```python
from build123d import *

# Parameters (mm, degrees)
CYLINDER024_R               = 7.5
CYLINDER024_DEPTH           = 2
CYLINDER012_R               = 3.15
CYLINDER012_DEPTH           = 43
CYLINDER011_R               = 2
CYLINDER011_DEPTH           = 39
CYLINDER013_R               = 2.55
CYLINDER013_DEPTH           = 6
BOX022_W                    = 1
BOX022_H                    = 7
BOX022_DEPTH                = 4
BOX023_W                    = 1
BOX023_H                    = 7
BOX023_DEPTH                = 4
CHAMFER003068012002016_SIZE = 3
BOX020_W                    = 7.8
BOX020_H                    = 3
BOX020_DEPTH                = 1
BOX018_W                    = 7.8
BOX018_H                    = 7
BOX018_DEPTH                = 1
BOX021_W                    = 5
BOX021_H                    = 4
BOX021_DEPTH                = 5
CHAMFER003068012002041_SIZE = 3
CHAMFER003068012002042_SIZE = 0.4
BOX017_W                    = 25
BOX017_H                    = 5
BOX017_DEPTH                = 24
CHAMFER003068012002002_SIZE = 4
BOX015_W                    = 24
BOX015_H                    = 20
BOX015_DEPTH                = 38
CHAMFER003068012002006_SIZE = 2
CHAMFER003068012002007_SIZE = 2
CHAMFER003068012002009_SIZE = 0.4
CYLINDER023_R               = 6
CYLINDER023_DEPTH           = 27
CHAMFER003068012002044_SIZE = 0.4
CHAMFER003068012002045_SIZE = 0.4


with BuildPart() as cylinder024:
    # Cylinder024 → Cylinder024 (new body)
    with BuildSketch(Plane(origin=(-15, 6, -12), x_dir=(1, 0, 0), z_dir=(0, 0, 1))):
        Circle(CYLINDER024_R)
    extrude(amount=CYLINDER024_DEPTH)


with BuildPart() as cylinder012:
    # Cylinder012 → Cylinder012 (new body)
    with BuildSketch(Plane(origin=(-15, 6, -11), x_dir=(1, 0, 0), z_dir=(0, 0, 1))):
        Circle(CYLINDER012_R)
    extrude(amount=CYLINDER012_DEPTH)


with BuildPart() as cylinder011:
    # Cylinder011 → Cylinder011 (new body)
    with BuildSketch(Plane(origin=(1, 13, -5), x_dir=(0, 0, 1), z_dir=(-1, 0, 0))):
        Circle(CYLINDER011_R)
    extrude(amount=CYLINDER011_DEPTH)


with BuildPart() as fusion001002012005:
    # Cylinder013 → Cylinder013 (new body)
    with BuildSketch(Plane(origin=(1, 13, -5), x_dir=(0, 0, 1), z_dir=(-1, 0, 0))):
        Circle(CYLINDER013_R)
    extrude(amount=CYLINDER013_DEPTH)

    # Fusion001002012005: union Cylinder011
    add(cylinder011.part)


with BuildPart() as cube022:
    # Box022 → Box022 (new body)
    with BuildSketch(Plane(origin=(-2.5, 0.5, 16.5), x_dir=(1, 0, 0), z_dir=(0, 0, 1))):
        with Locations((0.5, 3.5)):
            Rectangle(BOX022_W, BOX022_H)
    extrude(amount=BOX022_DEPTH)


with BuildPart() as chamfer003068012002016:
    # Box023 → Box023 (new body)
    with BuildSketch(Plane(origin=(-2.5, 0.5, 11), x_dir=(1, 0, 0), z_dir=(0, 0, 1))):
        with Locations((0.5, 3.5)):
            Rectangle(BOX023_W, BOX023_H)
    extrude(amount=BOX023_DEPTH)

    # Fusion001002012009: union Cube022
    add(cube022.part)

    # Chamfer003068012002016
    chamfer003068012002016_edges = [chamfer003068012002016.edges().sort_by_distance(p)[0] for p in [
        (-2, 0.5, 11),
        (-2, 7.5, 11),
        (-2, 0.5, 20.5),
        (-2, 7.5, 20.5),
    ]]
    chamfer(chamfer003068012002016_edges, length=CHAMFER003068012002016_SIZE)


with BuildPart() as chamfer003068012002016_1:
    # Chamfer003068012002016 placement: moved
    add(chamfer003068012002016.part.moved(Location((0, 0, 1.5))))


with BuildPart() as cube020:
    # Box020 → Box020 (new body)
    with BuildSketch(Plane(origin=(-18.9, -2, 28), x_dir=(1, 0, 0), z_dir=(0, 0, 1))):
        with Locations((3.9, 1.5)):
            Rectangle(BOX020_W, BOX020_H)
    extrude(amount=BOX020_DEPTH)


with BuildPart() as fusion001002012023:
    # Box018 → Box018 (new body)
    with BuildSketch(Plane(origin=(-18.9, 11, 28), x_dir=(1, 0, 0), z_dir=(0, 0, 1))):
        with Locations((3.9, 3.5)):
            Rectangle(BOX018_W, BOX018_H)
    extrude(amount=BOX018_DEPTH)

    # Fusion001002012023: union Cube020
    add(cube020.part)


with BuildPart() as chamfer003068012002042:
    # Box021 → Box021 (new body)
    with BuildSketch(Plane(origin=(-26, -5, -5), x_dir=(1, 0, 0), z_dir=(0, 0, 1))):
        with Locations((2.5, 2)):
            Rectangle(BOX021_W, BOX021_H)
    extrude(amount=BOX021_DEPTH)

    # Chamfer003068012002041
    chamfer003068012002041_edges = [chamfer003068012002042.edges().sort_by_distance(p)[0] for p in [
        (-23.5, -5, -5),
    ]]
    chamfer(chamfer003068012002041_edges, length=CHAMFER003068012002041_SIZE)

    # Chamfer003068012002042
    chamfer003068012002042_edges = [chamfer003068012002042.edges().sort_by_distance(p)[0] for p in [
        (-26, -5, -1),
        (-26, -3.5, -3.5),
        (-26, -3, 0),
        (-21, -5, -1),
        (-21, -3.5, -3.5),
        (-21, -3, 0),
    ]]
    chamfer(chamfer003068012002042_edges, length=CHAMFER003068012002042_SIZE)


with BuildPart() as chamfer003068012002002:
    # Box017 → Box017 (new body)
    with BuildSketch(Plane(origin=(-26, 11, 2), x_dir=(1, 0, 0), z_dir=(0, 0, 1))):
        with Locations((12.5, 2.5)):
            Rectangle(BOX017_W, BOX017_H)
    extrude(amount=BOX017_DEPTH)

    # Chamfer003068012002002
    chamfer003068012002002_edges = [chamfer003068012002002.edges().sort_by_distance(p)[0] for p in [
        (-13.5, 11, 2),
        (-13.5, 11, 26),
    ]]
    chamfer(chamfer003068012002002_edges, length=CHAMFER003068012002002_SIZE)


with BuildPart() as chamfer003068012002009:
    # Box015 → Box015 (new body)
    with BuildSketch(Plane(origin=(-26, -2, -10), x_dir=(1, 0, 0), z_dir=(0, 0, 1))):
        with Locations((12, 10)):
            Rectangle(BOX015_W, BOX015_H)
    extrude(amount=BOX015_DEPTH)

    # Cut001008: cut Chamfer003068012002002
    add(chamfer003068012002002.part, mode=Mode.SUBTRACT)

    # Chamfer003068012002006
    chamfer003068012002006_edges = [chamfer003068012002009.edges().sort_by_distance(p)[0] for p in [
        (-14, 18, -10),
    ]]
    chamfer(chamfer003068012002006_edges, length=CHAMFER003068012002006_SIZE)

    # Chamfer003068012002007
    chamfer003068012002007_edges = [chamfer003068012002009.edges().sort_by_distance(p)[0] for p in [
        (-14, -2, -10),
    ]]
    chamfer(chamfer003068012002007_edges, length=CHAMFER003068012002007_SIZE)

    # Chamfer003068012002009
    chamfer003068012002009_edges = [chamfer003068012002009.edges().sort_by_distance(p)[0] for p in [
        (-26, 8, -10),
        (-26, -1, -9),
        (-26, 17, -9),
        (-26, -2, 10),
        (-26, 18, 10),
        (-26, 13, 4),
        (-26, 15.5, 2),
        (-26, 16, 14),
        (-26, 15.5, 26),
        (-26, 13, 24),
        (-26, 11, 14),
        (-2, 8, -10),
        (-2, -1, -9),
        (-2, 17, -9),
        (-2, -2, 10),
        (-2, 18, 10),
        (-2, 13, 4),
        (-2, 15.5, 2),
        (-2, 16, 14),
        (-2, 15.5, 26),
        (-2, 13, 24),
        (-2, 11, 14),
    ]]
    chamfer(chamfer003068012002009_edges, length=CHAMFER003068012002009_SIZE)


with BuildPart() as universal_pulley_mount:
    # Cylinder023 → Cylinder023 (new body)
    with BuildSketch(Plane(origin=(1, 13, -5), x_dir=(0, 0, 1), z_dir=(-1, 0, 0))):
        Circle(CYLINDER023_R)
    extrude(amount=CYLINDER023_DEPTH)

    # Chamfer003068012002044
    chamfer003068012002044_edges = [universal_pulley_mount.edges().sort_by_distance(p)[0] for p in [
        (-26, 13, -11),
    ]]
    chamfer(chamfer003068012002044_edges, length=CHAMFER003068012002044_SIZE)

    # Fusion001002012022: union Chamfer003068012002009
    add(chamfer003068012002009.part)

    # Fusion001002012024: union Fusion001002012023, Chamfer003068012002042
    add(fusion001002012023.part)
    add(chamfer003068012002042.part)

    # Cut001023: cut Chamfer003068012002016
    add(chamfer003068012002016_1.part, mode=Mode.SUBTRACT)

    # Cut001024: cut Fusion001002012005
    add(fusion001002012005.part, mode=Mode.SUBTRACT)

    # Cut001025: cut Cylinder012
    add(cylinder012.part, mode=Mode.SUBTRACT)

    # Cut001026: cut Cylinder024
    add(cylinder024.part, mode=Mode.SUBTRACT)

    # Chamfer003068012002045
    chamfer003068012002045_edges = [universal_pulley_mount.edges().sort_by_distance(p)[0] for p in [
        (1, 13, -11),
        (1, 13, -7.55),
        (-18.15, 6, -10),
        (-26, 13, -7),
    ]]
    chamfer(chamfer003068012002045_edges, length=CHAMFER003068012002045_SIZE)


solid = universal_pulley_mount.part
```
Can you work these out from the model? Positions are in its coordinate system, mm. A direction names the side the tool comes from. Give positions to 0.01 mm unless a question says otherwise; leave off trailing zeros. Loops run counter-clockwise (first coordinate to the right, second up) from the corner with the lowest first, then second, coordinate; pieces in that order, holes last. Notation, with made-up numbers: M 54.5,-38.5 L 100.5,-38.5 A8 cw 100.5,-32.5 Z; hole C 39.5,-5.5 d2. An arc over 180 degrees is marked long. Use one line per item in the form item = value. Start each with the question number.
(1) I want a section at C-C, the plane y = 6. Write out the boundary of the cut face in (x, z).
(2) Thinking about a two-plate mould opening in Z: for faces 1 (the flat face through (-24, -3, -4)), 2 (the flat face through (-15, 0, 29)), 3 (the flat face through (-14, 11, 14)), which applies, released by +Z, released by -Z, zero draft, split by the parting line, or undercut?
(3) Please list where these lines run through material, in increasing order: line 1 (Y direction, x = -15, z = 3.5); line 2 (Y direction, x = -15, z = 14); line 3 (Z direction, x = -2.5, y = 12).
(4) I want a section at D-D, the plane x = -15. Write out the boundary of the cut face in (y, z), and give its area (3 significant figures).
(5) On a 3-axis mill with a long thin cutter (end or side, diameter ignored), from which of +Z, -Z, +X, -X, +Y, -Y can I reach the whole of each face in a straight line? I mean faces 4 (the flat face through (-24, -3, 0)), 5 (the flat face through (-14, 13, 24)), 6 (the flat face through (-14, 18, 13)), 7 (the flat face through (-2.5, 4, 15)). Say none if no direction works.
(6) I'm going to push flat-ended pins straight in: P1, Ø2, axis at x = -12.5, z = 1, coming from the -Y side; P2, Ø2, axis at x = -14.5, z = 23, coming from the +Y side; P3, Ø12, axis at y = 5, z = 21.5, coming from the +X side. Where does each tip first touch, or does it pass through?
(7) I want a section at B-B, the plane x = -3.75. Write out the boundary of the cut face in (y, z).
(8) I want a section at A-A, the plane z = 17.5. Write out the boundary of the cut face in (x, y).
Worked out:
q1.outline = M -26,-9.6 L -25.6,-10 L -18.55,-10 L -18.15,-9.6 L -18.15,28 L -26,28 Z; M -11.85,-9.6 L -11.45,-10 L -2.4,-10 L -2,-9.6 L -2,14 L -2.5,14 L -2.5,16.5 L -2,16.5 L -2,18 L -2.5,18 L -2.5,20.5 L -2,20.5 L -2,28 L -11.85,28 Z
q2.face_1 = released by -Z
q2.face_2 = released by +Z
q2.face_3 = undercut
q3.line_1 = -2 to 2.85, 9.15 to 13.5, 16 to 18
q3.line_2 = -2 to 2.85, 9.15 to 11, 16 to 18
q3.line_3 = -10.92 to -7.35, -2.65 to 5, 23 to 28
q4.outline = M -2,-8 L 0,-10 L 2.45,-10 L 2.85,-9.6 L 2.85,28 L 1,28 L 1,29 L -2,29 Z; M 9.15,-9.6 L 9.55,-10 L 13.5,-10 L 13.5,-10.98 A6 ccw 18,-1.68 L 18,29 L 11,29 L 11,28 L 9.15,28 Z; hole C 13,-5 d4; hole M 11,6 L 15,2 L 16,2 L 16,26 L 15,26 L 11,22 Z
q4.area = 417 mm²
q5.face_4 = +Z, +X, -X, -Y
q5.face_5 = +X, -X
q5.face_6 = +Z, +X, -X, +Y
q5.face_7 = +X
q6.P1 = -2
q6.P2 = 18
q6.P3 = -2
q7.outline = M -2,-8 L 0,-10 L 9.68,-10 A6 ccw 18,-1.68 L 18,28 L -2,28 Z; hole C 13,-5 d5.1; hole M 11,6 L 15,2 L 16,2 L 16,26 L 15,26 L 11,22 Z
q8.outline = M -26,-1.6 L -25.6,-2 L -2.4,-2 L -2,-1.6 L -2,10.6 L -2.4,11 L -25.6,11 L -26,10.6 Z; M -26,16.4 L -25.6,16 L -2.4,16 L -2,16.4 L -2,17.6 L -2.4,18 L -25.6,18 L -26,17.6 Z; hole C -15,6 d6.3
